Verification items for the finished model (mm, model axes). Face numbers are marked on the shaded views. Give positions to 0.01 mm unless a question says otherwise; leave off trailing zeros. Order: outer loops, then holes, each group sorted by start corner. A loop starts at its lowest first (then second) coordinate and runs counter-clockwise, first axis right, second up. Notation, with made-up numbers: M 2.5,17.25 L 6.5,17.25 A24 ccw 6.5,53.25 Z; hole C -9.75,13.5 d10. An arc over 180 degrees is marked long. Answer as a JSON object with one key per item and string values.
```python
from build123d import *

# Parameters (mm, degrees)
F1_DEPTH  = 79.248
F3_DEPTH  = 11.2522
F6_R      = 3.175
F6_R_2    = 25.273
F6_R_3    = 21.209
F7_DEPTH  = 7.62
F9_R      = 4.191
F10_DEPTH = 7.874


# Not quite as in the source:
# - ends of sketch curves that miss each other by under 0.0002 mm in the source are joined
# - a feature names something its author has since deleted; it is built from what else it names


with BuildPart() as f1:
    # F0 (on Front) → F1 (new body)
    with BuildSketch(Plane.XZ):
        with BuildLine():
            ThreePointArc((25.2730608729, 1.6496396764), (17.870749032, 19.5203708791), (0, 26.9226396763))
            ThreePointArc((0, 26.9226396763), (-17.8706272863, -16.2210915263), (25.2730608729, 1.6496396764))
        make_face()
        with BuildLine():
            ThreePointArc((0, 24.3826396763), (14.9970630949, 18.1706867446), (21.2090547187, 3.1736396764))
            ThreePointArc((21.2090547187, 3.1736396764), (-14.9969536575, -11.8234073918), (0, 24.3826396763))
        make_face(mode=Mode.SUBTRACT)
    extrude(amount=-F1_DEPTH)

    # F2 (on face) → F3 (cut)
    with BuildSketch(Plane.XZ):
        with BuildLine():
            Line((24.13, 26.9226396763), (0, 26.9226396763))
            ThreePointArc((0, 26.9226396763), (8.7356829544, 25.3648971249), (16.3944827501, 20.8836579854))
            Line((16.3944827501, 20.8836579854), (24.13, 20.8835978808))
            Line((24.13, 20.8835978808), (24.13, 26.9226396763))
        make_face()
        with BuildLine():
            ThreePointArc((-16.3944315191, 20.8835978808), (-8.7356618013, 25.3648600709), (0, 26.9226396763))
            Line((0, 26.9226396763), (-24.13, 26.9226396763))
            Line((-24.13, 26.9226396763), (-24.13, 20.8835978808))
            Line((-24.13, 20.8835978808), (-16.3944315191, 20.8835978808))
        make_face()
    extrude(amount=-F3_DEPTH, mode=Mode.SUBTRACT)

    # F4 (on Right) → F5 (revolve)
    with BuildSketch(Plane.YZ):
        Polygon((1.143, 28.0148396764), (0, 26.9226396764), (3.0988, 26.9226396764), (3.0988, 28.0148396764), align=None)
        Polygon((8.0772, 28.0148396764), (3.0988, 26.9226396764), (8.0772, 26.9226396764), align=None)
    revolve(axis=Axis((6.08729e-05, 0, 1.6496396764), (0, 1, 0)))

    # F6 (on face) → F7 (join)
    with BuildSketch(Plane(origin=(0, 79.248, 0), x_dir=(-1, 0, 0), z_dir=(0, 1, 0))):
        with BuildLine():
            Line((-25.1332705243, -33.6252276427), (25.6667294757, -33.6252276427))
            ThreePointArc((25.6667294757, -33.6252276427), (32.8509343726, -30.6494325395), (35.8267294757, -23.4652276427))
            Line((35.8267294757, -23.4652276427), (35.8267294757, 27.3347723573))
            ThreePointArc((35.8267294757, 27.3347723573), (32.8509343726, 34.5189772542), (25.6667294757, 37.4947723573))
            Line((25.6667294757, 37.4947723573), (-25.1332705243, 37.4947723573))
            ThreePointArc((-25.1332705243, 37.4947723573), (-32.3174754212, 34.5189772542), (-35.2932705243, 27.3347723573))
            Line((-35.2932705243, 27.3347723573), (-35.2932705243, -23.4652276427))
            ThreePointArc((-35.2932705243, -23.4652276427), (-32.3174754212, -30.6494325395), (-25.1332705243, -33.6252276427))
        make_face()
        with Locations((-25.1332705243, -23.4652276427)):
            Circle(F6_R, mode=Mode.SUBTRACT)
        with Locations((-6.08729e-05, 1.6496396764)):
            Circle(F6_R_2, mode=Mode.SUBTRACT)
        with Locations((25.6667294757, -23.4652276427)):
            Circle(F6_R, mode=Mode.SUBTRACT)
        with Locations((-25.1332705243, 27.3347723573)):
            Circle(F6_R, mode=Mode.SUBTRACT)
        with Locations((25.6667294757, 27.3347723573)):
            Circle(F6_R, mode=Mode.SUBTRACT)
        with Locations((-6.08729e-05, 1.6496396764)):
            Circle(F6_R_2)
        with Locations((-5.47187e-05, 3.1736396764)):
            Circle(F6_R_3, mode=Mode.SUBTRACT)
    extrude(amount=-F7_DEPTH)

    # F9 (on offset) → F10 (cut)
    with BuildSketch(Plane.XY.offset(28.448)):
        with Locations((4.8756e-06, 26.1899903387)):
            Circle(F9_R)
    extrude(amount=-F10_DEPTH, mode=Mode.SUBTRACT)


solid = f1.part
```
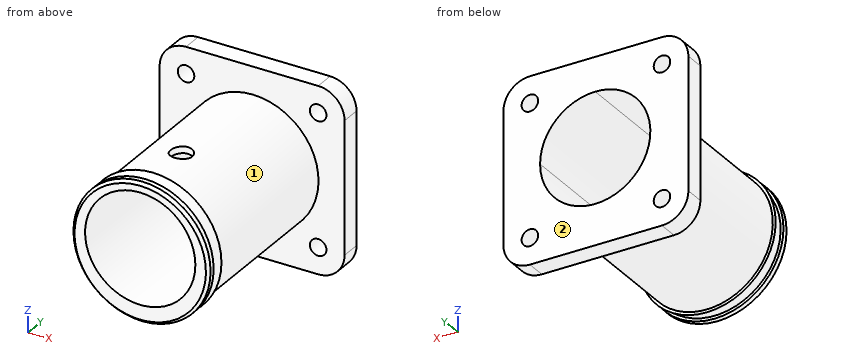
Q1. Section check C-C on x = -2. Count the separate pieces of the cut face and the enclosed holes in it, then the cut area to 3 significant figures.
Resolved:
{"separate pieces": "3", "enclosed holes": "0", "area": "797 mm²"}
Q2. Section check B-B on y = 42.5. Record the cut outline in (x, z), then the cut area to 3 significant figures.
Resolved:
{"outline": "C 0,1.65 d50.55; hole C 0,3.17 d42.42", "area": "593 mm²"}
Q3. Section check A-A on y = 74. Record the cut outline in (x, z) (3 decimals), then the cut area to 3 significant figures.
Resolved:
{"outline": "M -35.827,-23.465 A10.16 ccw -25.667,-33.625 L 25.133,-33.625 A10.16 ccw 35.293,-23.465 L 35.293,27.335 A10.16 ccw 25.133,37.495 L -25.667,37.495 A10.16 ccw -35.827,27.335 Z; hole C -25.667,-23.465 d6.35; hole C -25.667,27.335 d6.35; hole C 0,3.174 d42.418; hole C 25.133,-23.465 d6.35; hole C 25.133,27.335 d6.35", "area": "3,430 mm²"}
Q4. Gauge pin test, flat ends, axial feed: pin 1 Ø6.5 at (x, y) = (0, 26.19) entering from +Z; pin 2 Ø7.5 at (x, z) = (-25.67, -23.47) entering from -Y; pin 3 Ø3 at (y, z) = (48.5, 5.5) entering from +X. Record the tip position at first contact, or that the pin passes through.
Resolved:
{"pin 1": "stops at z = -17.78", "pin 2": "stops at y = 71.63", "pin 3": "stops at x = 25.16"}
Q5. Section check D-D on y = 24. Record the cut outline in (x, z), then the cut area to 3 significant figures.
Resolved:
{"outline": "M -3.57,24.08 L -3.57,26.67 A25.27 ccw long 3.57,26.67 L 3.57,24.08 A21.21 cw long Z", "area": "575 mm²"}
Q6. Release check for a two-part mould opening along Y. For the marked faces 1 and 2 record: +Y half, -Y half, draft (parallel to the pull), parting line (faces both ways), or undercut.
Resolved:
{"face 1": "undercut", "face 2": "+Y half"}
Q7. Material ranges on L1, parallel to Y at x = -16.5, z = -21; L2, parallel to X at y = 15, z = 15; L3, parallel to X at y = 7, z = -6, recorded low to high.
Resolved:
{"L1": "y = 71.63 to 79.25", "L2": "x = -21.46 to -17.61, 17.61 to 21.46", "L3": "x = -24.98 to -19.12, 19.12 to 24.98"}
